from build123d import *

# Parameters (mm, degrees)
SKETCH_1_R      = 1.5
SKETCH_1_R_2    = 4.25
EXTRUDE_1_DEPTH = 1


with BuildPart() as part:
    # 草图1 → 凸台-拉伸1 (new body)
    with BuildSketch(Plane.XY):
        with BuildLine():
            Line((-10.070213397, 30.026651359), (-3.9, 9.129214461))
            ThreePointArc((-3.9, 9.129214461), (-4.497287215, 5.649388777), (-7.618135885, 3.998255109))
            ThreePointArc((-7.618135885, 3.998255109), (-10.871519118, -2.152407684), (-3.922863507, -1.789998466))
            Line((-3.922863507, -1.789998466), (-3.251614082, -0.448572281))
            ThreePointArc((-3.251614082, -0.448572281), (0, 1.560317266), (3.251614082, -0.448572281))
            Line((3.251614082, -0.448572281), (3.922863507, -1.789998466))
            ThreePointArc((3.922863507, -1.789998466), (10.871519118, -2.152407684), (7.618135885, 3.998255109))
            ThreePointArc((7.618135885, 3.998255109), (4.497287215, 5.649388777), (3.9, 9.129214461))
            Line((3.9, 9.129214461), (10.070213397, 30.026651359))
            ThreePointArc((10.070213397, 30.026651359), (0, 43.5), (-10.070213397, 30.026651359))
        make_face()
        with Locations((-7.5, 0)):
            Circle(SKETCH_1_R, mode=Mode.SUBTRACT)
        with Locations((7.5, 0)):
            Circle(SKETCH_1_R, mode=Mode.SUBTRACT)
        with Locations((0, 33)):
            Circle(SKETCH_1_R_2, mode=Mode.SUBTRACT)
        with Locations((0, 40.25)):
            Circle(SKETCH_1_R, mode=Mode.SUBTRACT)
        with Locations((-7.25, 33)):
            Circle(SKETCH_1_R, mode=Mode.SUBTRACT)
        with Locations((0, 25.75)):
            Circle(SKETCH_1_R, mode=Mode.SUBTRACT)
        with Locations((7.25, 33)):
            Circle(SKETCH_1_R, mode=Mode.SUBTRACT)
        with BuildLine():
            Line((-5.112098998, 23.828498278), (-1.022796172, 9.978742645))
            ThreePointArc((-1.022796172, 9.978742645), (0, 9.214287127), (1.022796172, 9.978742645))
            Line((1.022796172, 9.978742645), (5.112098998, 23.828498278))
            ThreePointArc((5.112098998, 23.828498278), (0, 22.5), (-5.112098998, 23.828498278))
        make_face(mode=Mode.SUBTRACT)
    extrude(amount=EXTRUDE_1_DEPTH)


solid = part.part
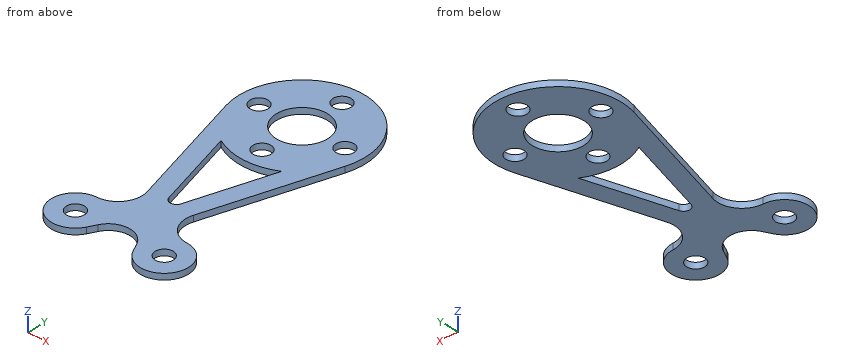
Model file for the job. Use its own axes, mm. Give positions to 0.01 mm unless a question says otherwise; leave off trailing zeros. Order: outer loops, then holes, each group sorted by start corner. A loop starts at its lowest first (then second) coordinate and runs counter-clockwise, first axis right, second up. Notation, with made-up numbers: M -10,-3 L 21,-3 A14 cw 21,9 Z; hole C -23.5,-17.75 d7. An arc over 180 degrees is marked long. Put each result on its own line as item: value. Start each with the question number.
(1) Drill centre lines: L1, parallel to X at y = 12, z = 0.2; L2, parallel to X at y = 15.5, z = 0.35. Where is each one in solid material? Low to high. Write a range as [from, to].
(2) Band-saw the part on A-A on z = 0.4. Count the separate pieces of the cut face and the enclosed holes in it, then the cut area to 3 significant figures.
(3) Pin check, flat tips, straight feed: pin 1 Ø3.5 at (x, y) = (0, 40.25) entering from -Z; pin 2 Ø1.8 at (x, y) = (-7.5, 0) entering from +Z. Stop position of each tip, or through.
(4) Band-saw the part on B-B on x = 0. Give the cut face in (y, z), then the cut area to 3 significant figures.
(5) Band-saw the part on C-C on y = 23. Give the cut face in (x, z).
(6) Band-saw the part on D-D on y = 40.25. Give the cut face in (x, z), then the cut area to 3 significant figures.
Results below:
1. L1: x = [-4.75, -1.62], [1.62, 4.75]
1. L2: x = [-5.78, -2.65], [2.65, 5.78]
2. separate pieces: 1
2. enclosed holes: 8
2. area: 525 mm2
3. pin 1: stops at z = 0
3. pin 2: passes through
4. outline: M 1.56,0 L 9.21,0 L 9.21,1 L 1.56,1 Z; M 22.5,0 L 24.25,0 L 24.25,1 L 22.5,1 Z; M 27.25,0 L 28.75,0 L 28.75,1 L 27.25,1 Z; M 37.25,0 L 38.75,0 L 38.75,1 L 37.25,1 Z; M 41.75,0 L 43.5,0 L 43.5,1 L 41.75,1 Z
4. area: 14.2 mm2
5. outline: M -8,0 L -4.87,0 L -4.87,1 L -8,1 Z; M -3.2,0 L 3.2,0 L 3.2,1 L -3.2,1 Z; M 4.87,0 L 8,0 L 8,1 L 4.87,1 Z
6. outline: M -7.6,0 L -1.5,0 L -1.5,1 L -7.6,1 Z; M 1.5,0 L 7.6,0 L 7.6,1 L 1.5,1 Z
6. area: 12.2 mm2
